The listing builds one solid part. Answer for the finished solid, in the listing's coordinates (mm). Give positions to 0.01 mm unless a question says otherwise; leave off trailing zeros. Order: outer loops, then holes, each group sorted by start corner. A loop starts at its lowest first (then second) coordinate and runs counter-clockwise, first axis right, second up. Notation, with made-up numbers: (37.25, -37) - (91.25, -37) arc R9 ccw to (91.25, -32) - close; hole circle Ø10 at (-22.75, 48.5). An arc over 180 degrees is marked (long way). Use a Markdown table: item, result. Add a question column.
1) Flat-ended cylindrical pins translate along their axes: pin 1 (2 mm diameter, centred on x = -33.5, y = -0.5, fed in from +Z); pin 2 (2.5 mm diameter, centred on x = -16, z = -233, fed in from +Y); pin 3 (3.5 mm diameter, centred on x = -9.57, z = -117.07, fed in from +Y); pin 4 (1.6 mm diameter, centred on y = 1, z = -219.5, fed in from +X) (3 decimals). Find the tip coordinate at first contact, or state that the pin passes through.
2) Find section C-C, the plane z = -45. Determine the outline of the cut face in (x, y), plus the area to 3 significant figures.
3) Find section A-A, the plane y = 1.2. Determine the outline of the cut face in (x, z) (3 decimals).
4) Straight lines are drawn through the part: line 1 (Z direction, x = 0, y = -0.9); line 2 (Z direction, x = -13.5, y = -1.65); line 3 (Z direction, x = 29, y = -0.9). For each, find the intervals that lie inside material, in ascending order.
5) Find section B-B, the plane z = -179. Determine the outline of the cut face in (x, y), plus the area to 3 significant figures.
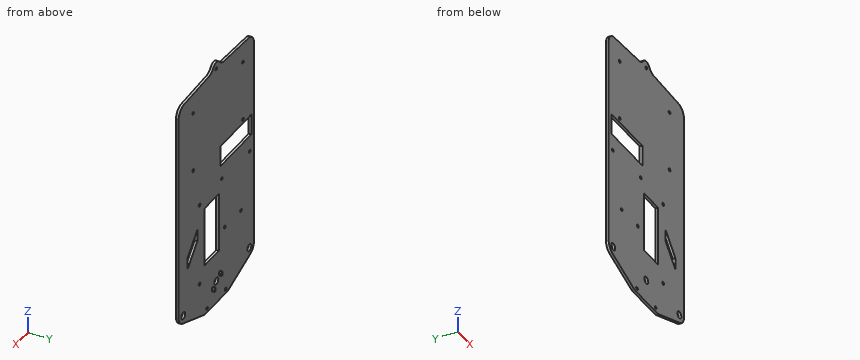
Autodesk Inventor part; units mm, degrees
ref_plane "YZ Plane" through (0, 0, 0) normal (1, 0, 0) x (0, 1, 0)
ref_plane "XZ Plane" through (0, 0, 0) normal (0, 1, 0) x (-1, 0, 0)
ref_plane "XY Plane" through (0, 0, 0) normal (0, 0, 1) x (1, 0, 0)
sketch "Sketch2" plane through (0, 0, 0) normal (0, 1, 0) x (-1, 0, 0)
  line L0 (60, -21.0659) -> (-26, -21.0659) construction
  line L1 (-26, -21.0659) -> (-26, -79.0659) construction
  line L2 (-26, -79.0659) -> (60, -79.0659) construction
  line L3 (60, -79.0659) -> (60, -21.0659) construction
  line L4 (-41.5, -22.5659) -> (-60.5, -22.5659) construction
  line L5 (-60.5, -22.5659) -> (-60.5, -78.5659) construction
  line L6 (-60.5, -78.5659) -> (-41.5, -78.5659) construction
  line L7 (-41.5, -78.5659) -> (-41.5, -22.5659) construction
  line L8 (46, -21.0659) -> (-40, -21.0659) construction
  line L9 (-40, -21.0659) -> (-40, -79.0659) construction
  line L10 (-40, -79.0659) -> (46, -79.0659) construction
  line L11 (46, -79.0659) -> (46, -21.0659) construction
  line L12 (-29, -120.6366) -> (-29, -200.6366) construction
  line L13 (65, -3.0659) -> (65, -220.6213)
  line L14 (65, -220.6213) -> (20, -237)
  line L15 (20, -237) -> (-20, -237)
  line L16 (-20, -237) -> (-65, -220.6213)
  line L17 (-65, -220.6213) -> (-65, -3.0659)
  line L18 (65, -3.0659) -> (6.5, 0)
  line L19 (-65, -3.0659) -> (-6.5, 0)
  arc A0 (6.5, 0) -> (-6.5, 0) centre (0, 0) ccw
  line L20 (16, -233) -> (-16, -233) construction
  line L21 (6.5, 0) -> (-6.5, 0) construction
  line L22 (-32.8737, -143.5299) -> (-32.8737, -154.8521)
  line L23 (-32.8737, -154.8521) -> (-50, -173.5831)
  line L24 (-50, -173.5831) -> (-50, -162.2608)
  line L25 (-50, -162.2608) -> (-32.8737, -143.5299)
  line L26 (4.3202, -129.3254) -> (-20, -129.3254)
  line L27 (-20, -129.3254) -> (-20, -186.991)
  line L28 (-20, -186.991) -> (4.3202, -186.991)
  line L29 (4.3202, -186.991) -> (4.3202, -129.3254)
  line L30 (64, -4.0659) -> (-36, -4.0659) construction
  line L31 (-36, -4.0659) -> (-36, -83.0659) construction
  line L32 (-36, -83.0659) -> (64, -83.0659) construction
  line L33 (64, -83.0659) -> (64, -4.0659) construction
  line L34 (50, -4.0659) -> (-50, -4.0659) construction
  line L35 (-50, -4.0659) -> (-50, -83.0659) construction
  line L36 (-50, -83.0659) -> (50, -83.0659) construction
  line L37 (50, -83.0659) -> (50, -4.0659) construction
  line L38 (57, -215.6213) -> (-57, -215.6213) construction
  line L39 (42.5503, -169.1692) -> (14.6503, -169.1692) construction
  line L40 (60.3703, -103.0992) -> (7.0303, -103.0992) construction
  line L41 (7.0303, -103.0992) -> (7.0303, -204.6992) construction
  line L42 (7.0303, -204.6992) -> (60.3703, -204.6992) construction
  line L43 (60.3703, -204.6992) -> (60.3703, -103.0992) construction
  line L44 (60.3601, -82.95) -> (6.9778, -82.95)
  line L45 (6.9778, -82.95) -> (6.9778, -103.0146)
  line L46 (6.9778, -103.0146) -> (60.3601, -103.0146)
  line L47 (60.3601, -103.0146) -> (60.3601, -82.95)
  line L48 (6, -209.375) -> (6, -211.625) construction
  line L49 (4.875, -209.375) -> (4.875, -211.625)
  line L50 (7.125, -211.625) -> (7.125, -209.375)
  arc A1 (7.125, -209.375) -> (4.875, -209.375) centre (6, -209.375) ccw
  arc A2 (4.875, -211.625) -> (7.125, -211.625) centre (6, -211.625) ccw
  line L51 (-6, -218.375) -> (-6, -220.625) construction
  line L52 (-7.125, -218.375) -> (-7.125, -220.625)
  line L53 (-4.875, -220.625) -> (-4.875, -218.375)
  arc A3 (-4.875, -218.375) -> (-7.125, -218.375) centre (-6, -218.375) ccw
  arc A4 (-7.125, -220.625) -> (-4.875, -220.625) centre (-6, -220.625) ccw
  point P0 (0, -215)
  point P1 (57.7903, -118.3692)
  point P2 (9.5703, -117.0692)
  point P3 (6, -210.5)
  point P4 (-6, -219.5)
  dimension "d0" = 130
  dimension "d1" = 32
  dimension "d4" = 65
  dimension "d5" = 0
  dimension "d6" = 6.5
  dimension "d7" = 93
  dimension "d8" = 93
  dimension "d9" = 4
  dimension "d11" = 237
  dimension "d12" = 160
  dimension "d14" = 86
  dimension "d15" = 86
  dimension "d16" = 58
  dimension "d17" = 4
  dimension "d18" = 4
  dimension "d19" = 4
  dimension "d20" = 100
  dimension "d21" = 100
  dimension "d22" = 79
  dimension "d23" = 50
  dimension "d24" = 19
  dimension "d25" = 56
  dimension "d26" = 15.5
  dimension "d27" = 1.5
  dimension "d28" = 40
  dimension "d29" = 20
  dimension "d30" = 4
  dimension "d31" = 160
  dimension "d32" = 80
  dimension "d33" = 36
  dimension "d34" = 0
  dimension "d35" = 22
  dimension "d36" = 1
  dimension "d37" = 1
  dimension "d38" = 27.9
  dimension "d39" = 1.3
  dimension "d40" = 50.8
  dimension "d41" = 15.24
  dimension "d42" = 5.08
  dimension "d43" = 13.97
  dimension "d44" = 101.6
  dimension "d45" = 2.54
  dimension "d46" = 53.34
  dimension "d78" = 8
  dimension "d79" = 8
  dimension "d80" = 5
  dimension "d81" = 2.25
  dimension "d82" = 2.25
  dimension "d83" = 2.25
  dimension "d84" = 2.25
  dimension "d85" = 12
  dimension "d86" = 6
  dimension "d87" = 9
  dimension "d88" = 4.5
extrude "Extrusion1" add sketch "Sketch2" against normal blind 2.5 contours L13 L14 L15 L16 L17 L19 A0 L18 | A1 L50 A2 L49 | A3 L53 A4 L52
hole "Hole1" at (0, 0, 0) at (-16, 0, -233) at (16, 0, -233) at (29, 0, -120.6366) at (29, 0, -200.6366) at (-57.7903, 0, -118.3692) at (-9.5703, 0, -117.0692) at (-14.6503, 0, -169.1692) at (-42.5503, 0, -169.1692) direction (0, -1, 0) diameter 2.8956 depth 2.5
hole "Hole2" at (-57, 0, -215.6213) at (0, 0, -215) at (57, 0, -215.6213) direction (0, -1, 0) diameter 6.756 depth 2.5
hole "Jetson-only" at (-46, 0, -21.0659) at (-46, 0, -79.0659) at (40, 0, -79.0659) at (40, 0, -21.0659) direction (0, -1, 0) diameter 2.8956 depth 2.5
hole "Jetson + PCA 9685" [suppressed]
fillet "Fillet1" radius 10 8 edges at (-65, -1.25, -220.6213) (-20, -1.25, -237) (20, -1.25, -237) (65, -1.25, -220.6213) (65, -1.25, -3.0659) (6.5, -1.25, 0) (-6.5, -1.25, 0) (-65, -1.25, -3.0659)
extrude "Extrusion2" add sketch "Sketch2" along normal blind 2 contours A1 L50 A2 L49 | A3 L53 A4 L52
equation "\"d17\" = d18"
equation "\"d19\" = d17"
equation "\"d21\" = d20"
properties part number "chassis_plate_v7"
The answers:
| question | item | result |
|---|---|---|
| 1 | pin 1 | z = -1.36 |
| 1 | pin 2 | through |
| 1 | pin 3 | y = 0 |
| 1 | pin 4 | x = 7.125 |
| 2 | outline | (-65, -2.5) - (65, -2.5) - (65, 0) - (-65, 0) - close |
| 2 | area | 325 mm2 |
| 3 | outline | (-7.125, -211.625) arc R1.125 ccw to (-4.875, -211.625) - (-4.875, -209.375) arc R1.125 ccw to (-7.125, -209.375) - close; (4.875, -220.625) arc R1.125 ccw to (7.125, -220.625) - (7.125, -218.375) arc R1.125 ccw to (4.875, -218.375) - close |
| 4 | line 1 | -237 to -218.38, -211.62 to -186.99, -129.33 to -1.45, 1.45 to 6.5 |
| 4 | line 2 | -237 to -170.05, -168.29 to -103.01, -82.95 to -0.37 |
| 4 | line 3 | -233.72 to -202.08, -199.19 to -122.08, -119.19 to -1.18 |
| 5 | outline | (-65, -2.5) - (-4.32, -2.5) - (-4.32, 0) - (-65, 0) - close; (20, -2.5) - (65, -2.5) - (65, 0) - (20, 0) - close |
| 5 | area | 264 mm2 |
